from build123d import *

# Parameters (mm, degrees)
SKETCH1_W           = 44.85
SKETCH1_H           = 44.85
SKETCH1_W_2         = 38.5
SKETCH1_H_2         = 38.5
BOSS_EXTRUDE1_DEPTH = 19.25
SKETCH2_W           = 44.85
SKETCH2_H           = 44.85
BOSS_EXTRUDE2_DEPTH = 3.175
SKETCH3_W           = 44.85
SKETCH3_H           = 44.85
BOSS_EXTRUDE3_DEPTH = 3.175
SKETCH5_R           = 12.7
CUT_EXTRUDE1_DEPTH  = 3.175
CUT_EXTRUDE2_START  = 22.425
SKETCH6_R           = 10
CUT_EXTRUDE2_DEPTH  = 41.675
SKETCH7_R           = 12.7
CUT_EXTRUDE3_DEPTH  = 55.929807482
SKETCH8_W           = 44.85
SKETCH8_H           = 44.85
SKETCH8_R           = 2.2225
BOSS_EXTRUDE4_DEPTH = 6.35
SKETCH9_R           = 3.4925
CUT_EXTRUDE4_DEPTH  = 6.35
CUT_EXTRUDE5_REACH  = 62.226
SKETCH10_W          = 38.5
SKETCH10_H          = 38.5
SKETCH11_R          = 12.1285
BOSS_EXTRUDE5_DEPTH = 25.4


with BuildPart() as part:
    # Sketch1 → Boss-Extrude1 (new, symmetric)
    with BuildSketch(Plane(origin=(0, 0, 0), x_dir=(1, 0, 0), z_dir=(0, 1, 0))):
        Rectangle(SKETCH1_W, SKETCH1_H)
        Rectangle(SKETCH1_W_2, SKETCH1_H_2, mode=Mode.SUBTRACT)
    extrude(amount=BOSS_EXTRUDE1_DEPTH, both=True)

    # Sketch2 → Boss-Extrude2 (add)
    with BuildSketch(Plane(origin=(0, 19.25, 0), x_dir=(1, 0, 0), z_dir=(0, 1, 0))):
        Rectangle(SKETCH2_W, SKETCH2_H)
    extrude(amount=BOSS_EXTRUDE2_DEPTH)

    # Sketch3 → Boss-Extrude3 (add)
    with BuildSketch(Plane.XZ.offset(19.25)):
        Rectangle(SKETCH3_W, SKETCH3_H)
    extrude(amount=BOSS_EXTRUDE3_DEPTH)

    # Sketch5 → Cut-Extrude1 (cut)
    with BuildSketch(Plane(origin=(0, -22.425, -22.425), x_dir=(1, 0, 0), z_dir=(0, 1, 0))):
        with Locations(Location((0, -22.425, 0), (0, 0, 90))):
            Circle(SKETCH5_R)
    extrude(amount=CUT_EXTRUDE1_DEPTH, mode=Mode.SUBTRACT)

    # Sketch6 → Cut-Extrude2 (cut)
    with BuildSketch(Plane(origin=(0, 0, 0), x_dir=(1, 0, 0), z_dir=(0, 1, 0)).offset(CUT_EXTRUDE2_START)):
        with Locations(Location((0, 0, 0), (0, 0, 270))):
            Circle(SKETCH6_R)
    extrude(amount=-CUT_EXTRUDE2_DEPTH, mode=Mode.SUBTRACT)

    # Sketch7 → Cut-Extrude3 (cut, through all)
    with BuildSketch(Plane.ZY.offset(22.425)):
        Circle(SKETCH7_R)
    extrude(amount=-CUT_EXTRUDE3_DEPTH, mode=Mode.SUBTRACT)

    # Sketch8 → Boss-Extrude4 (add)
    with BuildSketch(Plane(origin=(0, 0, -22.425), x_dir=(-1, 0, 0), z_dir=(0, 0, -1))):
        Rectangle(SKETCH8_W, SKETCH8_H)
        with Locations((-12.7, 12.7)):
            Circle(SKETCH8_R, mode=Mode.SUBTRACT)
        with Locations((0, 12.7)):
            Circle(SKETCH8_R, mode=Mode.SUBTRACT)
        with Locations((12.7, 12.7)):
            Circle(SKETCH8_R, mode=Mode.SUBTRACT)
        Circle(SKETCH8_R, mode=Mode.SUBTRACT)
        with Locations((12.7, 0)):
            Circle(SKETCH8_R, mode=Mode.SUBTRACT)
        with Locations((0, -12.7)):
            Circle(SKETCH8_R, mode=Mode.SUBTRACT)
        with Locations((12.7, -12.7)):
            Circle(SKETCH8_R, mode=Mode.SUBTRACT)
        with Locations((-12.7, 0)):
            Circle(SKETCH8_R, mode=Mode.SUBTRACT)
        with Locations((-12.7, -12.7)):
            Circle(SKETCH8_R, mode=Mode.SUBTRACT)
    extrude(amount=BOSS_EXTRUDE4_DEPTH)

    # Sketch9 → Cut-Extrude4 (cut)
    with BuildSketch(Plane.XY.offset(-19.25)):
        with Locations((12.7, 12.7)):
            Circle(SKETCH9_R)
        with Locations((0, 12.7)):
            Circle(SKETCH9_R)
        with Locations((-12.7, 12.7)):
            Circle(SKETCH9_R)
        Circle(SKETCH9_R)
        with Locations((-12.7, 0)):
            Circle(SKETCH9_R)
        with Locations((0, -12.7)):
            Circle(SKETCH9_R)
        with Locations((-12.7, -12.7)):
            Circle(SKETCH9_R)
        with Locations((12.7, 0)):
            Circle(SKETCH9_R)
        with Locations((12.7, -12.7)):
            Circle(SKETCH9_R)
    extrude(amount=-CUT_EXTRUDE4_DEPTH, mode=Mode.SUBTRACT)

    # Sketch10 → Cut-Extrude5 (cut, up to next)
    with BuildSketch(Plane.XY.offset(22.425), mode=Mode.PRIVATE) as cut_extrude5_sk1:
        Rectangle(SKETCH10_W, SKETCH10_H)
    cut_extrude5_tool1 = extrude(cut_extrude5_sk1.sketch, amount=-CUT_EXTRUDE5_REACH, mode=Mode.PRIVATE) & part.part
    add(cut_extrude5_tool1.solids().sort_by_distance((0, 0, 22.425))[0], mode=Mode.SUBTRACT)

    # Sketch11 → Boss-Extrude5 (add)
    with BuildSketch(Plane(origin=(0, 22.425, 0), x_dir=(1, 0, 0), z_dir=(0, 1, 0))):
        with BuildLine():
            Line((-15.3035, 0), (-15.3035, 28.775))
            Line((-15.3035, 28.775), (15.3035, 28.775))
            Line((15.3035, 28.775), (15.3035, 0))
            ThreePointArc((15.3035, 0), (0, -15.3035), (-15.3035, 0))
        make_face()
        with Locations(Location((0, 0, 0), (0, 0, 270))):
            Circle(SKETCH11_R, mode=Mode.SUBTRACT)
    extrude(amount=BOSS_EXTRUDE5_DEPTH)


solid = part.part
Can you work these out from the model? Positions are in its coordinate system, mm. A direction names the side the tool comes from. Coordinates: 2 decimals unless noted, no trailing zeros. Loops run counter-clockwise (first coordinate to the right, second up) from the corner with the lowest first, then second, coordinate; pieces in that order, holes last. Notation, with made-up numbers: (-11.5, -1.5) - (16.5, -1.5) arc R23 ccw to (16.5, 21.5) - close; hole circle Ø6 at (55, -17.5). An arc over 180 degrees is marked (long way). Answer as a JSON object with one key per item and string values. Group by question number.
Item 1: If we section it at B-B (x = 13.5): State how many separate pieces and enclosed holes the cut face has, plus the area to 3 significant figures.
Item 2: If we section it at A-A (y = 37.5): List the corners of the cut face in (x, z) for me (1 decimal), plus the area to 3 significant figures.
Item 3: If we mould it in two halves opening along Z, with no side actions, what happens to faces 4 (the face through (-13, 10, -25.6)), 5 (the face through (19.25, -9, 11)), 6 (the face through (7.7, -20.9, 10.1))? For each: released by +Z, released by -Z, zero draft, split by the parting line, or undercut.
Item 4: On a 3-axis mill with a long thin cutter (end or side, diameter ignored), from which of +Z, -Z, +X, -X, +Y, -Y can I reach the whole of each face in a straight line? I mean faces 1 (the face through (0.3, 34.9, 15.3)), 2 (the face through (20.82, -12.4, -2.75)), 3 (the face through (0.7, -2.3, -25.6)). Say none if no direction works.
Item 5: If we section it at C-C (y = 17.5): List the corners of the cut face in (x, z) for me (3 decimals).
Item 6: If I drill on L1, parallel to Y at x = -12.7, z = -27.65 (1 decimal); L2, parallel to X at y = 16.5, z = -9 (3 decimals); L3, parallel to X at y = 21, z = 0 (3 decimals), over which ranges is the centre line in solid material (lowest first)? Write a range as from..to.
Item 7: For pin 1 (8 mm diameter, centred on y = 23.5, z = -9.5, fed in from -X) (3 decimals); pin 2 (4 mm diameter, centred on x = -9, z = -2, fed in from +Y) (3 decimals); pin 3 (5.5 mm diameter, centred on x = -1.5, y = -13, fed in from +Z); pin 4 (2 mm diameter, centred on x = -14.5, y = 11.5, fed in from +Z), each with a flat end and sliding along its axis, tell me the tip position at first contact or that it passes through.
Returned:
{
 "1": {"separate pieces": "4", "enclosed holes": "0", "area": "1,440 mm²"},
 "2": {"outline": "(-15.3, -28.8) - (15.3, -28.8) - (15.3, 0) arc R15.3 ccw to (-15.3, 0) - close; hole circle Ø24.3 at (0, 0)", "area": "786 mm²"},
 "3": {"face 4": "released by +Z", "face 5": "zero draft", "face 6": "undercut"},
 "4": {"face 1": "+Z, +Y", "face 2": "+X, -X", "face 3": "+Z"},
 "5": {"outline": "(-22.425, -28.775) - (22.425, -28.775) - (22.425, 22.425) - (19.25, 22.425) - (19.25, -19.25) - (-19.25, -19.25) - (-19.25, 22.425) - (-22.425, 22.425) - close"},
 "6": {"L1": "y = -22.4..-14.9, -10.5..-2.2, 2.2..10.5, 14.9..47.8", "L2": "x = -22.425..-19.25, 19.25..22.425", "L3": "x = -22.425..-10, 10..22.425"},
 "7": {"pin 1": "stops at x = -22.425", "pin 2": "stops at y = 22.425", "pin 3": "stops at z = -19.25", "pin 4": "stops at z = -25.6"}
}
